The model under review builds one solid part; all positions refer to its coordinate system, in mm. Face numbers are marked on the shaded views. Coordinates: 2 decimals unless noted, no trailing zeros. Order: outer loops, then holes, each group sorted by start corner. A loop starts at its lowest first (then second) coordinate and runs counter-clockwise, first axis right, second up. Notation, with made-up numbers: (26.25, -0.75) - (48.25, -0.75) arc R5 ccw to (48.25, 4.25) - close; hole circle Ø3 at (61.5, -38). An arc over 180 degrees is marked (long way). Answer in a Markdown table with one row per item.
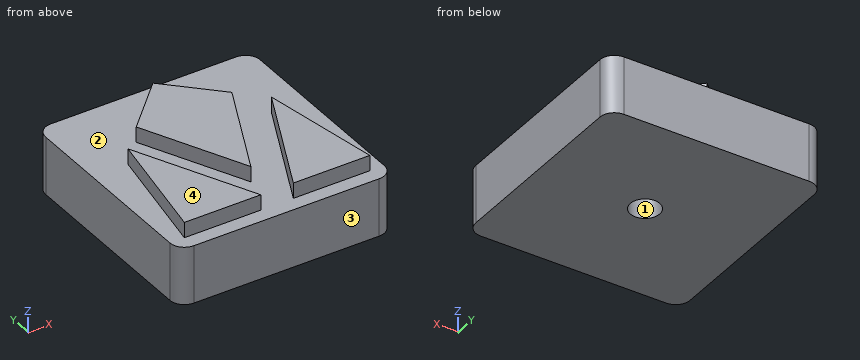
```python
from build123d import *

# Parameters (mm, degrees)
F1_DEPTH = 10
F2_DEPTH = 12.67
F4_D     = 5.1054
F4_DEPTH = 10
F4_TIP   = 1.5338169022
F5_R     = 2.5


with BuildPart() as f1:
    # F0 (on Top) → F1 (new body)
    with BuildSketch(Plane.XY):
        Polygon((-8.2773605124, 24.7226394876), (0, 33), (8.2773605124, 24.7226394876), (12.4160407685, 20.5839592315), (18.5455481509, 14.4544518491), (18.5455481509, 35.5), (-18.5455481509, 35.5), (-18.5455481509, 14.4544518491), (-12.4160407685, 20.5839592315), align=None)
        Polygon((0, 0), (-2.8175829438, 0), (-16.0455481509, 0), (-18.5455481509, 0), (-18.5455481509, -2.5), (18.5455481509, -2.5), (18.5455481509, 0), (16.0455481509, 0), (2.8175829438, 0), align=None)
        Polygon((-16.0455481509, 0), (-12.4160407685, 20.5839592315), (-18.5455481509, 14.4544518491), (-18.5455481509, 0), align=None)
        Polygon((-2.8175829438, 0), (-12.4160407685, 20.5839592315), (-16.0455481509, 0), align=None)
        Polygon((0, 6.9717825853), (-8.2773605124, 24.7226394876), (-12.4160407685, 20.5839592315), (-2.8175829438, 0), (0, 0), (2.8175829438, 0), (12.4160407685, 20.5839592315), (8.2773605124, 24.7226394876), align=None)
        Polygon((16.0455481509, 0), (12.4160407685, 20.5839592315), (2.8175829438, 0), align=None)
        Polygon((18.5455481509, 14.4544518491), (12.4160407685, 20.5839592315), (16.0455481509, 0), (18.5455481509, 0), align=None)
        Polygon((8.2773605124, 24.7226394876), (0, 33), (-8.2773605124, 24.7226394876), (0, 6.9717825853), align=None)
    extrude(amount=F1_DEPTH)

    # F0 (on Top) → F2 (join)
    with BuildSketch(Plane.XY):
        Polygon((16.0455481509, 0), (12.4160407685, 20.5839592315), (2.8175829438, 0), align=None)
        Polygon((8.2773605124, 24.7226394876), (0, 33), (-8.2773605124, 24.7226394876), (0, 6.9717825853), align=None)
        Polygon((-2.8175829438, 0), (-12.4160407685, 20.5839592315), (-16.0455481509, 0), align=None)
    extrude(amount=F2_DEPTH)

    # F4
    with Locations(Plane(origin=(0, 0, 0), x_dir=(1, 0, 0), z_dir=(0, 0, -1))):
        with Locations((0, -16.5)):
            Hole(F4_D / 2, depth=F4_DEPTH)
            with Locations((0, 0, -(F4_DEPTH + F4_TIP / 2))):  # 118° drill point
                Cone(0, F4_D / 2, F4_TIP, mode=Mode.SUBTRACT)

    # F5
    f5_edges = [f1.edges().sort_by_distance(p)[0] for p in [
        (-18.545548, 35.5, 5),
        (18.545548, 35.5, 5),
        (18.545548, -2.5, 5),
        (-18.545548, -2.5, 5),
    ]]
    fillet(f5_edges, radius=F5_R)


solid = f1.part
```
Item 1: We need section C-C, the plane y = 27. Write out the cut boundary in (x, z).
Check values:
| item | result |
|---|---|
| outline | (-18.55, 0) - (18.55, 0) - (18.55, 10) - (6, 10) - (6, 12.67) - (-6, 12.67) - (-6, 10) - (-18.55, 10) - close |
Item 2: Clearance check with flat-ended pins moving along their axes: pin 1 Ø3 at (y, z) = (28, 10.5) entering from +X; pin 2 Ø1.5 at (x, y) = (6.5, 19) entering from +Z; pin 3 Ø0.8 at (x, z) = (-10.5, 11) entering from -Y. State where each tip first meets the part, or that it passes through.
Check values:
| item | result |
|---|---|
| pin 1 | x = 18.55 |
| pin 2 | z = 10 |
| pin 3 | y = 0 |
Item 3: We need section D-D, the plane x = 15. Write out the cut boundary in (y, z), then the cut area to 3 significant figures.
Check values:
| item | result |
|---|---|
| outline | (-2.5, 0) - (35.5, 0) - (35.5, 10) - (5.93, 10) - (5.93, 12.67) - (0, 12.67) - (0, 10) - (-2.5, 10) - close |
| area | 396 mm^2 |
Item 4: We need section B-B, the plane z = 3. Write out the cut boundary in (x, y).
Check values:
| item | result |
|---|---|
| outline | (-18.55, 0) arc R2.5 ccw to (-16.05, -2.5) - (16.05, -2.5) arc R2.5 ccw to (18.55, 0) - (18.55, 33) arc R2.5 ccw to (16.05, 35.5) - (-16.05, 35.5) arc R2.5 ccw to (-18.55, 33) - close; hole circle Ø5.11 at (0, 16.5) |
Item 5: Mouldability with a two-part tool opening along Y and no side actions: class the marked faces 1, 2, 3 and 4 as +Y half, -Y half, draft (parallel to the pull), parting line (faces both ways), or undercut.
Check values:
| item | result |
|---|---|
| face 1 | undercut |
| face 2 | undercut |
| face 3 | -Y half |
| face 4 | draft |
Item 6: To check wall thickness, follow line 1 (X direction, y = 16.5, z = 4.5); line 2 (Y direction, x = 0, z = 7); line 3 (Z direction, x = 12.5, y = 30). State the ranges of each line that lie inside material, in increasing order. Write a range as from..to.
Check values:
| item | result |
|---|---|
| line 1 | -18.55..-2.55, 2.55..18.55 |
| line 2 | -2.5..13.95, 19.05..35.5 |
| line 3 | 0..10 |
Item 7: We need section A-A, the plane z = 10.5. Write out the cut boundary in (x, y).
Check values:
| item | result |
|---|---|
| outline | (-16.05, 0) - (-2.82, 0) - (-12.42, 20.58) - close; (-8.28, 24.72) - (0, 6.97) - (8.28, 24.72) - (0, 33) - close; (2.82, 0) - (16.05, 0) - (12.42, 20.58) - close; hole circle Ø3.44 at (0, 16.5) |
